Check sheet for the drawn part. Datum: minimum x, y, z corner. Units: mm. A direction names the side the tool comes from. Give positions to 0.01 mm unless a question says otherwise; leave off trailing zeros. Loops run counter-clockwise (first coordinate to the right, second up) from the corner with the lowest first, then second, coordinate; pieces in that order, holes last. Notation, with made-up numbers: (23.5, 13.5) -> (81.5, 13.5) arc R9 cw to (81.5, 29.5) -> close; hole circle Ø10 at (22.25, 23.25). An arc over 180 degrees is marked (long way). One line per question, with ' | ' between items.
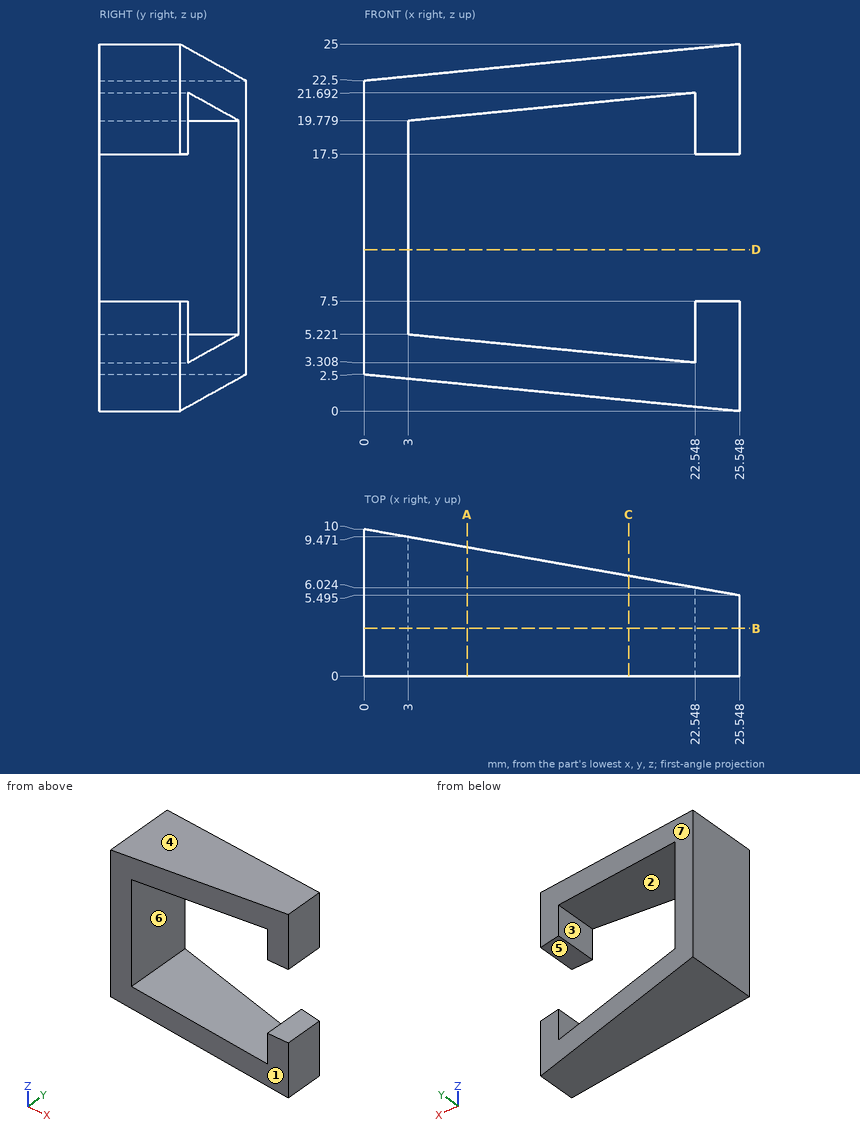
Item 1: Set-up check for the marked faces 5, 6 and 7: record each of +Z, -Z, +X, -X, +Y, -Y from which the full face is reachable in a straight line by a thin tool's end or side.
Result:
face 5: +X, +Y, -Y | face 6: +Y, -Y | face 7: +Z, -Z, +X, +Y
Item 2: Scan lines: probe 1 along X at (y, z) = (3.75, 6.5); probe 2 along X at (y, z) = (1, 10.5); probe 3 along Z at (x, y) = (18.75, 5.75) (1 decimal). Record each from-to range of solid material in increasing order.
Result:
probe 1: 0 to 3, 22.55 to 25.55 | probe 2: 0 to 3 | probe 3: 0.7 to 3.7, 21.3 to 24.3
Item 3: Sectioned sample at A-A (x = 7). Record the cut outline in (y, z) (1 decimal).
Result:
outline: (0, 1.8) -> (8.8, 1.8) -> (8.8, 4.8) -> (0, 4.8) -> close; (0, 20.2) -> (8.8, 20.2) -> (8.8, 23.2) -> (0, 23.2) -> close
Item 4: Release check for a two-part mould opening along Z. For the marked faces 1, 2, 3 and 4 record: pulls with the +Z half, pulls with the -Z half, needs draft (parallel to the pull), parting line crosses it, or undercut.
Result:
face 1: needs draft | face 2: undercut | face 3: undercut | face 4: pulls with the +Z half
Item 5: Sectioned sample at B-B (y = 3.25). Record the cut outline in (x, z), plus the area to 3 significant figures.
Result:
outline: (0, 2.5) -> (25.55, 0) -> (25.55, 7.5) -> (22.55, 7.5) -> (22.55, 3.31) -> (3, 5.22) -> (3, 19.78) -> (22.55, 21.69) -> (22.55, 17.5) -> (25.55, 17.5) -> (25.55, 25) -> (0, 22.5) -> close | area: 223 mm2
Item 6: Sectioned sample at C-C (x = 18). Record the cut outline in (y, z).
Result:
outline: (0, 0.74) -> (6.83, 0.74) -> (6.83, 3.75) -> (0, 3.75) -> close; (0, 21.25) -> (6.83, 21.25) -> (6.83, 24.26) -> (0, 24.26) -> close
Item 7: Depth check by flat-ended pin: pin 1 Ø2.5 at (x, y) = (24, 3) entering from -Z; pin 2 Ø6 at (x, z) = (9, 22.5) entering from +Y; pin 3 Ø12 at (x, z) = (19.5, 14) entering from +Y; pin 4 Ø1.5 at (x, z) = (18, 19) entering from +Y. Enter the tip coordinate at first touch or a pass-through.
Result:
pin 1: z = 0.03 | pin 2: y = 8.94 | pin 3: y = 6.02 | pin 4: through
Item 8: Sectioned sample at D-D (z = 11). Record the cut outline in (x, y).
Result:
outline: (0, 0) -> (3, 0) -> (3, 9.47) -> (0, 10) -> close
